from build123d import *

# Parameters (mm, degrees)
BOSS_EXTRUDE1_DEPTH = 406.4
SKETCH2_W           = 317.5
SKETCH2_H           = 158.75
CUT_EXTRUDE1_DEPTH  = 114.3
CUT_EXTRUDE2_REACH  = 598.9
CUT_EXTRUDE3_REACH  = 598.9
SKETCH4_W           = 76.2
SKETCH4_H           = 88.9
CUT_EXTRUDE5_DEPTH  = 597.9


with BuildPart() as part:
    # Sketch1 → Boss-Extrude1 (new body)
    with BuildSketch(Plane(origin=(0, 0, 0), x_dir=(1, 0, 0), z_dir=(0, 1, 0))):
        Polygon((0, 0), (0, 241.3), (6.35, 241.3), (6.35, 6.35), (298.45, 6.35), (298.45, -101.6), (514.35, -101.6), (514.35, -38.1), (590.55, -38.1), (590.55, 241.3), (596.9, 241.3), (596.9, -44.45), (520.7, -44.45), (520.7, -107.95), (292.1, -107.95), (292.1, 0), align=None)
    extrude(amount=BOSS_EXTRUDE1_DEPTH)

    # Sketch2 → Cut-Extrude1 (cut)
    with BuildSketch(Plane.XY.offset(107.95)):
        with Locations((165.1, 79.375)):
            Rectangle(SKETCH2_W, SKETCH2_H)
    extrude(amount=-CUT_EXTRUDE1_DEPTH, mode=Mode.SUBTRACT)

    # Sketch3 → Cut-Extrude2 (cut, up to next)
    with BuildSketch(Plane.ZY, mode=Mode.PRIVATE) as cut_extrude2_sk1:
        Polygon((-76.2, 88.9), (-76.2, 139.7), (0, 139.7), (0, 0), (-241.3, 0), (-241.3, 88.9), align=None)
    cut_extrude2_tool1 = extrude(cut_extrude2_sk1.sketch, amount=-CUT_EXTRUDE2_REACH, mode=Mode.PRIVATE) & part.part
    add(cut_extrude2_tool1.solids().sort_by_distance((0, 55.127707, -108.030892))[0], mode=Mode.SUBTRACT)

    # Sketch4 → Cut-Extrude3 (cut, up to next)
    with BuildSketch(Plane(origin=(596.9, 0, 0), x_dir=(0, 0, -1), z_dir=(1, 0, 0)), mode=Mode.PRIVATE) as cut_extrude3_sk1:
        with Locations((203.2, 44.45)):
            Rectangle(SKETCH4_W, SKETCH4_H)
    cut_extrude3_tool1 = extrude(cut_extrude3_sk1.sketch, amount=-CUT_EXTRUDE3_REACH, mode=Mode.PRIVATE) & part.part
    add(cut_extrude3_tool1.solids().sort_by_distance((596.9, 44.45, -203.2))[0], mode=Mode.SUBTRACT)

    # Sketch6 → Cut-Extrude5 (cut, through all)
    with BuildSketch(Plane.ZY):
        Polygon((-241.3, 292.1), (-203.2, 292.1), (-139.7, 190.5), (-241.3, 190.5), align=None)
        Polygon((-88.9, 406.4), (-12.7, 406.4), (-12.7, 330.2), (-63.5, 330.2), align=None)
    extrude(amount=-CUT_EXTRUDE5_DEPTH, mode=Mode.SUBTRACT)


solid = part.part
Input: part model. Units: mm. Frame: model coordinates. A direction names the side the tool comes from. Give positions to 0.01 mm unless a question says otherwise; leave off trailing zeros. Loops run counter-clockwise (first coordinate to the right, second up) from the corner with the lowest first, then second, coordinate; pieces in that order, holes last. Notation, with made-up numbers: (62, 29) -> (121, 29) arc R8 ccw to (121, 44) -> close; hole circle Ø6 at (51.25, 36.5). An arc over 180 degrees is marked (long way). Answer as a JSON object with one key per item and string values. Group by question number.
Item 1: Cut plane D-D, the plane y = 54.5. Return the cut outline in (x, z).
Item 2: Reachability of faces 5 (the flat face through (514.35, 200, 70)), 6 (the flat face through (559, 200, 44.45)), 7 (the flat face through (3.131, 367.767, -76.022)) from +Z, -Z, +X, -X, +Y, -Y: full face, straight path, thin tool, end or side. Return the list, or none.
Item 3: Cut plane A-A, the plane y = 380. Return the cut outline in (x, z), and give its area (3 significant figures).
Item 4: Line query: probe 1 along X at (y, z) = (111, -165); probe 2 along X at (y, z) = (179.5, 38); probe 3 along Z at (x, y) = (294, 353). Output: solid intervals per line, ascending.
Item 5: Pull-direction query (X, two-part tool) for faces 1 (the flat face through (148, 301, 0)), 2 (the flat face through (6.35, 245, -119)), 3 (the flat face through (0, 245, -119)), 4 (the flat face through (298.45, 281, 47)); classes: released by +X, released by -X, zero draft, split by the parting line, or undercut.
Item 6: Pin query (flat end, axial travel): P1, Ø5, axis at y = 82.5, z = 104.5, coming from the -X side; P2, Ø1.9, axis at x = 592.5, y = 59.5, coming from the -Z side; P3, Ø12, axis at y = 128.5, z = -64, coming from the -X side. Return the tip coordinate at first contact, or that it passes through.
Item 7: Cut plane B-B, the plane y = 122.5. Return the cut outline in (x, z).
Item 8: Cut plane C-C, the plane x = 226.5. Return the cut outline in (y, z).
Checks:
{
 "1": {"outline": "(323.85, 101.6) -> (514.35, 101.6) -> (514.35, 38.1) -> (590.55, 38.1) -> (590.55, -165.1) -> (596.9, -165.1) -> (596.9, 44.45) -> (520.7, 44.45) -> (520.7, 107.95) -> (323.85, 107.95) -> close"},
 "2": {"face 5": "-Z, +Y, -Y", "face 6": "+Z, +X, +Y, -Y", "face 7": "+X, -X, +Y"},
 "3": {"outline": "(0, -241.3) -> (6.35, -241.3) -> (6.35, -80.1) -> (0, -80.1) -> close; (0, -12.7) -> (6.35, -12.7) -> (6.35, -6.35) -> (298.45, -6.35) -> (298.45, 101.6) -> (514.35, 101.6) -> (514.35, 38.1) -> (590.55, 38.1) -> (590.55, -12.7) -> (596.9, -12.7) -> (596.9, 44.45) -> (520.7, 44.45) -> (520.7, 107.95) -> (292.1, 107.95) -> (292.1, 0) -> (0, 0) -> close; (590.55, -241.3) -> (596.9, -241.3) -> (596.9, -80.1) -> (590.55, -80.1) -> close", "area": "7,290 mm²"},
 "4": {"probe 1": "x = 0 to 6.35, 590.55 to 596.9", "probe 2": "x = 292.1 to 298.45, 590.55 to 596.9", "probe 3": "z = -6.35 to 107.95"},
 "5": {"face 1": "zero draft", "face 2": "undercut", "face 3": "released by -X", "face 4": "undercut"},
 "6": {"P1": "stops at x = 323.85", "P2": "stops at z = -165.1", "P3": "stops at x = 590.55"},
 "7": {"outline": "(0, -241.3) -> (6.35, -241.3) -> (6.35, -76.2) -> (0, -76.2) -> close; (323.85, 101.6) -> (514.35, 101.6) -> (514.35, 38.1) -> (590.55, 38.1) -> (590.55, -241.3) -> (596.9, -241.3) -> (596.9, 44.45) -> (520.7, 44.45) -> (520.7, 107.95) -> (323.85, 107.95) -> close"},
 "8": {"outline": "(158.75, -6.35) -> (406.4, -6.35) -> (406.4, 0) -> (158.75, 0) -> close"}
}
